from build123d import *

# Parameters (mm, degrees)
SKETCH1_R           = 3.175
BOSS_EXTRUDE1_DEPTH = 5.08
SKETCH2_R           = 6.35
BOSS_EXTRUDE2_DEPTH = 3.175
SKETCH3_R           = 6.35
BOSS_EXTRUDE3_DEPTH = 3.175


with BuildPart() as part:
    # Sketch1 → Boss-Extrude1 (new body)
    with BuildSketch(Plane.XY):
        Circle(SKETCH1_R)
    extrude(amount=BOSS_EXTRUDE1_DEPTH)

    # Sketch2 → Boss-Extrude2 (add)
    with BuildSketch(Plane(origin=(0, 0, 0), x_dir=(-1, 0, 0), z_dir=(0, 0, -1))):
        Circle(SKETCH2_R)
    extrude(amount=BOSS_EXTRUDE2_DEPTH)

    # Sketch3 → Boss-Extrude3 (add)
    with BuildSketch(Plane.XY.offset(5.08)):
        Circle(SKETCH3_R)
    extrude(amount=BOSS_EXTRUDE3_DEPTH)


solid = part.part
Geometry: final body of the model. Coordinates: model frame, mm. A direction names the side the tool comes from. Round coordinates to 2 decimals unless told otherwise and drop trailing zeros. Loops run counter-clockwise (first coordinate to the right, second up) from the corner with the lowest first, then second, coordinate; pieces in that order, holes last. Notation, with made-up numbers: (-29.75, -21) - (13.25, -21) arc R33 cw to (13.25, 14) - close; hole circle Ø4 at (72, 33.25). An arc over 180 degrees is marked (long way). Write each question's results on one line, items separated by ' | '. Start each with the question number.
1) Cut plane A-A on y = -4.5. Return loops of the section in (x, z) (3 decimals).
2) Access query for faces 1 (the face through (-2, 3, 5.08)), 2 (the face through (1.38, -6.2, -1.57)). Directions: +Z, -Z, +X, -X, +Y, -Y. A direction counts if a zero-diameter tool reaches every point of the face in a straight line with its end or side. Return the directions, or none.
3) Cut plane C-C on x = 0. Return loops of the section in (y, z) (3 decimals).
4) Mould query, pull axis Z, two halves, no side actions, for faces 3 (the face through (-1.38, -6.2, 6.65)), 4 (the face through (0, 0, 8.255)), 5 (the face through (2, 3, 0)). Classes: released by +Z, released by -Z, zero draft, split by the parting line, or undercut.
5) First-contact query: P1, Ø6, axis at x = 4.5, z = 5, coming from the +Y side; P2, Ø3, axis at x = -1, z = 4.5, coming from the +Y side; P3, Ø5, axis at y = 3.5, z = 0.5, coming from the -X side; P4, Ø1.5, axis at y = 4, z = -1.5, coming from the -X side. Flat tips, straight axial feed; report the tip coordinate or a pass-through.
6) Line query: probe 1 along Z at (x, y) = (3.25, -2.5) (3 decimals); probe 2 along Y at (x, z) = (0, 3.25) (3 decimals); probe 3 along X at (y, z) = (3.25, -0.5). Output: solid intervals per line, ascending. Write a range as [from, to].
7) Cut plane B-B on x = 5.5. Return loops of the section in (y, z) (3 decimals).
Verdict:
1) outline: (-4.48, -3.175) - (4.48, -3.175) - (4.48, 0) - (-4.48, 0) - close; (-4.48, 5.08) - (4.48, 5.08) - (4.48, 8.255) - (-4.48, 8.255) - close
2) face 1: none | face 2: +Z, -Z
3) outline: (-6.35, -3.175) - (6.35, -3.175) - (6.35, 0) - (3.175, 0) - (3.175, 5.08) - (6.35, 5.08) - (6.35, 8.255) - (-6.35, 8.255) - (-6.35, 5.08) - (-3.175, 5.08) - (-3.175, 0) - (-6.35, 0) - close
4) face 3: zero draft | face 4: released by +Z | face 5: undercut
5) P1: stops at y = 6.17 | P2: stops at y = 6.35 | P3: stops at x = -6.26 | P4: stops at x = -5.46
6) probe 1: z = [-3.175, 0], [5.08, 8.255] | probe 2: y = [-3.175, 3.175] | probe 3: x = [-5.46, 5.46]
7) outline: (-3.174, -3.175) - (3.174, -3.175) - (3.174, 0) - (-3.174, 0) - close; (-3.174, 5.08) - (3.174, 5.08) - (3.174, 8.255) - (-3.174, 8.255) - close
